Here's how the part is built. I have some questions about the finished solid (model axes, mm). Coordinates: 2 decimals unless noted, no trailing zeros. Loops run counter-clockwise (first coordinate to the right, second up) from the corner with the lowest first, then second, coordinate; pieces in that order, holes last.
```python
from build123d import *

# Parameters (mm, degrees)
BOX011_W      = 4
BOX011_H      = 80
BOX011_DEPTH  = 4
FILLET006_R   = 1
BOX010_W      = 30
BOX010_H      = 4
BOX010_DEPTH  = 4
FILLET007_R   = 1
BOX009_W      = 30
BOX009_H      = 4
BOX009_DEPTH  = 4
FILLET008_R   = 1
BOX008_W      = 30
BOX008_H      = 4
BOX008_DEPTH  = 4
FILLET009_R   = 1
BOX013_W      = 4
BOX013_H      = 80
BOX013_DEPTH  = 4
FILLET010_R   = 1
BOX012_W      = 30
BOX012_H      = 4
BOX012_DEPTH  = 4
FILLET005_R   = 1
BOX006_W      = 45
BOX006_H      = 10
BOX006_DEPTH  = 10
BOX007_W      = 45
BOX007_H      = 10
BOX007_DEPTH  = 10
FILLET004_1_R = 2
FILLET004_2_R = 1
BOX003_W      = 116
BOX003_H      = 179.5
BOX003_DEPTH  = 20
FILLET002_R   = 1.5
BOX002_W      = 120
BOX002_H      = 181
BOX002_DEPTH  = 12
FILLET003_R   = 1.5
BOX001_W      = 98
BOX001_H      = 173.5
BOX001_DEPTH  = 4
FILLET_R      = 1.5
BOX_W         = 120
BOX_H         = 181
BOX_DEPTH     = 4
FILLET001_R   = 1.5


with BuildPart() as fillet006:
    # Box011 → Box011 (new body)
    with BuildSketch(Plane(origin=(0, 50, 5), x_dir=(1, 0, 0), z_dir=(0, 0, 1))):
        with Locations((2, 40)):
            Rectangle(BOX011_W, BOX011_H)
    extrude(amount=BOX011_DEPTH)

    # Fillet006
    fillet006_edges = [fillet006.edges().sort_by_distance(p)[0] for p in [
        (0, 50, 7),
        (0, 130, 7),
    ]]
    fillet(fillet006_edges, radius=FILLET006_R)


with BuildPart() as fillet007:
    # Box010 → Box010 (new body)
    with BuildSketch(Plane(origin=(85, -3.5, 5), x_dir=(1, 0, 0), z_dir=(0, 0, 1))):
        with Locations((15, 2)):
            Rectangle(BOX010_W, BOX010_H)
    extrude(amount=BOX010_DEPTH)

    # Fillet007
    fillet007_edges = [fillet007.edges().sort_by_distance(p)[0] for p in [
        (85, -3.5, 7),
        (115, -3.5, 7),
    ]]
    fillet(fillet007_edges, radius=FILLET007_R)


with BuildPart() as fillet008:
    # Box009 → Box009 (new body)
    with BuildSketch(Plane(origin=(4, 180.5, 5), x_dir=(1, 0, 0), z_dir=(0, 0, 1))):
        with Locations((15, 2)):
            Rectangle(BOX009_W, BOX009_H)
    extrude(amount=BOX009_DEPTH)

    # Fillet008
    fillet008_edges = [fillet008.edges().sort_by_distance(p)[0] for p in [
        (4, 184.5, 7),
        (34, 184.5, 7),
    ]]
    fillet(fillet008_edges, radius=FILLET008_R)


with BuildPart() as fillet009:
    # Box008 → Box008 (new body)
    with BuildSketch(Plane(origin=(85, 180.5, 5), x_dir=(1, 0, 0), z_dir=(0, 0, 1))):
        with Locations((15, 2)):
            Rectangle(BOX008_W, BOX008_H)
    extrude(amount=BOX008_DEPTH)

    # Fillet009
    fillet009_edges = [fillet009.edges().sort_by_distance(p)[0] for p in [
        (85, 184.5, 7),
        (115, 184.5, 7),
    ]]
    fillet(fillet009_edges, radius=FILLET009_R)


with BuildPart() as fillet010:
    # Box013 → Box013 (new body)
    with BuildSketch(Plane(origin=(120.5, 50, 5), x_dir=(1, 0, 0), z_dir=(0, 0, 1))):
        with Locations((2, 40)):
            Rectangle(BOX013_W, BOX013_H)
    extrude(amount=BOX013_DEPTH)

    # Fillet010
    fillet010_edges = [fillet010.edges().sort_by_distance(p)[0] for p in [
        (124.5, 50, 7),
        (124.5, 130, 7),
    ]]
    fillet(fillet010_edges, radius=FILLET010_R)


with BuildPart() as fusion002:
    # Box012 → Box012 (new body)
    with BuildSketch(Plane(origin=(4, -3.5, 5), x_dir=(1, 0, 0), z_dir=(0, 0, 1))):
        with Locations((15, 2)):
            Rectangle(BOX012_W, BOX012_H)
    extrude(amount=BOX012_DEPTH)

    # Fillet005
    fillet005_edges = [fusion002.edges().sort_by_distance(p)[0] for p in [
        (4, -3.5, 7),
        (34, -3.5, 7),
    ]]
    fillet(fillet005_edges, radius=FILLET005_R)

    # Fusion002: union Fillet006, Fillet007, Fillet008, Fillet009, Fillet010
    add(fillet006.part)
    add(fillet007.part)
    add(fillet008.part)
    add(fillet009.part)
    add(fillet010.part)


with BuildPart() as fusion002_1:
    # Fusion002 placement: moved
    add(fusion002.part.moved(Location((0, 0, 7))))


with BuildPart() as cube006:
    # Box006 → Box006 (new body)
    with BuildSketch(Plane(origin=(15, -5, 0), x_dir=(1, 0, 0), z_dir=(0, 0, 1))):
        with Locations((22.5, 5)):
            Rectangle(BOX006_W, BOX006_H)
    extrude(amount=BOX006_DEPTH)


with BuildPart() as fillet004:
    # Box007 → Box007 (new body)
    with BuildSketch(Plane(origin=(15, 175, 0), x_dir=(1, 0, 0), z_dir=(0, 0, 1))):
        with Locations((22.5, 5)):
            Rectangle(BOX007_W, BOX007_H)
    extrude(amount=BOX007_DEPTH)

    # Fusion: union Cube006
    add(cube006.part)


with BuildPart() as fillet004_1:
    # Fusion placement: moved
    add(fillet004.part.moved(Location((22, 0, 13))))

    # Fillet004 1
    fillet004_1_edges = [fillet004_1.edges().sort_by_distance(p)[0] for p in [
        (37, 180, 13),
        (82, 180, 13),
    ]]
    fillet(fillet004_1_edges, radius=FILLET004_1_R)

    # Fillet004 2
    fillet004_2_edges = [fillet004_1.edges().sort_by_distance(p)[0] for p in [
        (37, 0, 13),
        (82, 0, 13),
    ]]
    fillet(fillet004_2_edges, radius=FILLET004_2_R)


with BuildPart() as fillet002:
    # Box003 → Box003 (new body)
    with BuildSketch(Plane(origin=(4, 0.75, 4), x_dir=(1, 0, 0), z_dir=(0, 0, 1))):
        with Locations((58, 89.75)):
            Rectangle(BOX003_W, BOX003_H)
    extrude(amount=BOX003_DEPTH)

    # Fillet002
    fillet002_edges = [fillet002.edges().sort_by_distance(p)[0] for p in [
        (4, 0.75, 14),
        (4, 180.25, 14),
        (120, 0.75, 14),
        (120, 180.25, 14),
    ]]
    fillet(fillet002_edges, radius=FILLET002_R)


with BuildPart() as cut002:
    # Box002 → Box002 (new body)
    with BuildSketch(Plane(origin=(2, 0, 4), x_dir=(1, 0, 0), z_dir=(0, 0, 1))):
        with Locations((60, 90.5)):
            Rectangle(BOX002_W, BOX002_H)
    extrude(amount=BOX002_DEPTH)

    # Fillet003
    fillet003_edges = [cut002.edges().sort_by_distance(p)[0] for p in [
        (2, 0, 10),
        (2, 181, 10),
        (122, 0, 10),
        (122, 181, 10),
    ]]
    fillet(fillet003_edges, radius=FILLET003_R)

    # Cut001: cut Fillet002
    add(fillet002.part, mode=Mode.SUBTRACT)

    # Cut002: cut Fillet004
    add(fillet004_1.part, mode=Mode.SUBTRACT)


with BuildPart() as fillet_body:
    # Box001 → Box001 (new body)
    with BuildSketch(Plane(origin=(7, 4, 0), x_dir=(1, 0, 0), z_dir=(0, 0, 1))):
        with Locations((49, 86.75)):
            Rectangle(BOX001_W, BOX001_H)
    extrude(amount=BOX001_DEPTH)

    # Fillet
    fillet_edges = [fillet_body.edges().sort_by_distance(p)[0] for p in [
        (7, 4, 2),
        (7, 177.5, 2),
        (105, 4, 2),
        (105, 177.5, 2),
    ]]
    fillet(fillet_edges, radius=FILLET_R)


with BuildPart() as fusion003:
    # Box → Box (new body)
    with BuildSketch(Plane(origin=(2, 0, 0), x_dir=(1, 0, 0), z_dir=(0, 0, 1))):
        with Locations((60, 90.5)):
            Rectangle(BOX_W, BOX_H)
    extrude(amount=BOX_DEPTH)

    # Fillet001
    fillet001_edges = [fusion003.edges().sort_by_distance(p)[0] for p in [
        (2, 0, 2),
        (2, 181, 2),
        (122, 0, 2),
        (122, 181, 2),
    ]]
    fillet(fillet001_edges, radius=FILLET001_R)

    # Cut: cut Fillet body
    add(fillet_body.part, mode=Mode.SUBTRACT)

    # Fusion001: union Cut002
    add(cut002.part)

    # Fusion003: union Fusion002
    add(fusion002_1.part)


solid = fusion003.part
```
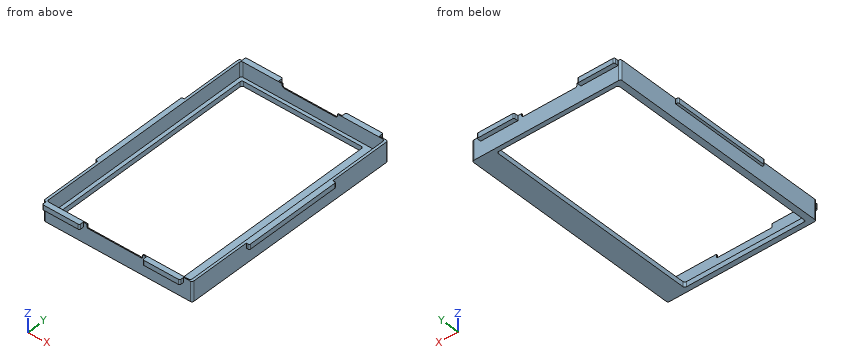
1. I want a section at B-B (y = 65). Please give me the cut outline in (x, z), then the cut area to 3 significant figures.
2. For pin 1 (1 mm diameter, centred on y = 103, z = 4, fed in from +X); pin 2 (5 mm diameter, centred on y = 29, z = 3, fed in from -X); pin 3 (2 mm diameter, centred on x = 94.5, z = 8, fed in from +Y), each with a flat end and sliding along its axis, tell me the tip position at first contact or that it passes through.
3. I need wall thicknesses on line 1 along X through (y, z) = (73.5, 9.5); line 2 along Y through (x, z) = (103, 4.75); line 3 along X through (y, z) = (20.5, 3). Which ranges of each line are inside material? Lowest first, please.
4. I want a section at A-A (x = 55). Please give me the cut outline in (y, z), then the cut area to 3 significant figures.
5. I want a section at C-C (z = 8). Please give me the cut outline in (x, y).
6. I want a section at D-D (x = 25.5). Please give me the cut outline in (y, z), then the cut area to 3 significant figures.
Response values:
1. outline: (0, 12) - (2, 12) - (2, 0) - (7, 0) - (7, 4) - (4, 4) - (4, 16) - (0, 16) - close; (105, 0) - (122, 0) - (122, 12) - (124.5, 12) - (124.5, 16) - (120, 16) - (120, 4) - (105, 4) - close
1. area: 154 mm2
2. pin 1: stops at x = 122
2. pin 2: stops at x = 2
2. pin 3: stops at y = 181
3. line 1: x = 2 to 4, 120 to 122
3. line 2: y = 0 to 0.75, 180.25 to 181
3. line 3: x = 2 to 7, 105 to 122
4. outline: (0, 0) - (4, 0) - (4, 4) - (0.75, 4) - (0.75, 13) - (0, 13) - close; (177.5, 0) - (181, 0) - (181, 13) - (180.25, 13) - (180.25, 4) - (177.5, 4) - close
4. area: 43.5 mm2
5. outline: (2, 1.5) arc R1.5 ccw to (3.5, 0) - (120.5, 0) arc R1.5 ccw to (122, 1.5) - (122, 179.5) arc R1.5 ccw to (120.5, 181) - (3.5, 181) arc R1.5 ccw to (2, 179.5) - close; hole (4, 2.25) arc R1.5 ccw to (5.5, 0.75) - (118.5, 0.75) arc R1.5 ccw to (120, 2.25) - (120, 178.75) arc R1.5 ccw to (118.5, 180.25) - (5.5, 180.25) arc R1.5 ccw to (4, 178.75) - close
6. outline: (-3.5, 12) - (0, 12) - (0, 0) - (4, 0) - (4, 4) - (0.75, 4) - (0.75, 16) - (-3.5, 16) - close; (177.5, 0) - (181, 0) - (181, 12) - (184.5, 12) - (184.5, 16) - (180.25, 16) - (180.25, 4) - (177.5, 4) - close
6. area: 76.0 mm2
